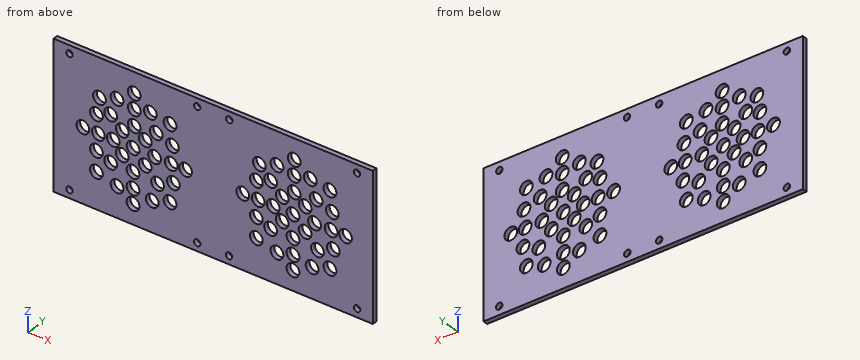
```python
from build123d import *

# Parameters (mm, degrees)
SKETCH1_W           = 200
SKETCH1_H           = 90
BOSS_EXTRUDE1_DEPTH = 3
SKETCH2_R           = 2
SKETCH2_R_2         = 4
CUT_EXTRUDE1_DEPTH  = 3


with BuildPart() as part:
    # Sketch1 → Boss-Extrude1 (new body)
    with BuildSketch(Plane(origin=(0, 0, 0), x_dir=(1, 0, 0), z_dir=(0, 1, 0))):
        with Locations((6.810810811, 7.918918919)):
            Rectangle(SKETCH1_W, SKETCH1_H)
    extrude(amount=BOSS_EXTRUDE1_DEPTH)

    # Sketch2 → Cut-Extrude1 (cut)
    with BuildSketch(Plane(origin=(0, 3, 0), x_dir=(1, 0, 0), z_dir=(0, 1, 0))):
        with Locations(Location((-83.189189189, 47.918918919, 0), (0, 0, 270))):
            Circle(SKETCH2_R)
        with Locations(Location((-83.189189189, -32.081081081, 0), (0, 0, 270))):
            Circle(SKETCH2_R)
        with Locations(Location((-3.189189189, 47.918918919, 0), (0, 0, 270))):
            Circle(SKETCH2_R)
        with Locations(Location((-3.189189189, -32.081081081, 0), (0, 0, 270))):
            Circle(SKETCH2_R)
        with Locations(Location((96.97523931, 47.753811706, 0), (0, 0, 270))):
            Circle(SKETCH2_R)
        with Locations(Location((96.890661701, -31.999841307, 0), (0, 0, 270))):
            Circle(SKETCH2_R)
        with Locations(Location((16.73095992, 47.837679145, 0), (0, 0, 270))):
            Circle(SKETCH2_R)
        with Locations(Location((16.92956487, -32.199971625, 0), (0, 0, 270))):
            Circle(SKETCH2_R)
        with Locations(Location((64.409536285, 15.225493569, 0), (0, 0, 270))):
            Circle(SKETCH2_R_2)
        with Locations(Location((64.458960542, 0.301508961, 0), (0, 0, 270))):
            Circle(SKETCH2_R_2)
        with Locations(Location((72.150575188, 22.957645887, 0), (0, 0, 270))):
            Circle(SKETCH2_R_2)
        with Locations(Location((79.984903702, 30.782980722, 0), (0, 0, 270))):
            Circle(SKETCH2_R_2)
        with Locations(Location((42.782150533, -6.377064303, 0), (0, 0, 270))):
            Circle(SKETCH2_R_2)
        with Locations(Location((35.744744462, -13.406391548, 0), (0, 0, 270))):
            Circle(SKETCH2_R_2)
        with Locations(Location((50.031602385, 0.251885254, 0), (0, 0, 270))):
            Circle(SKETCH2_R_2)
        with Locations(Location((71.328743505, -6.540662674, 0), (0, 0, 270))):
            Circle(SKETCH2_R_2)
        with Locations(Location((56.810810811, 7.918918919, 0), (0, 0, 270))):
            Circle(SKETCH2_R_2)
        with Locations(Location((79.984903702, -15.162031659, 0), (0, 0, 270))):
            Circle(SKETCH2_R_2)
        with Locations(Location((50.031602385, 14.670880058, 0), (0, 0, 270))):
            Circle(SKETCH2_R_2)
        with Locations(Location((42.782150533, 21.891194601, 0), (0, 0, 270))):
            Circle(SKETCH2_R_2)
        with Locations(Location((33.854481941, 30.782980722, 0), (0, 0, 270))):
            Circle(SKETCH2_R_2)
        with Locations(Location((70.286929504, 7.918918919, 0), (0, 0, 270))):
            Circle(SKETCH2_R_2)
        with Locations(Location((80.695917052, 7.918918919, 0), (0, 0, 270))):
            Circle(SKETCH2_R_2)
        with Locations(Location((89.69828466, 7.918918919, 0), (0, 0, 270))):
            Circle(SKETCH2_R_2)
        with Locations(Location((35.027656371, 7.918918919, 0), (0, 0, 270))):
            Circle(SKETCH2_R_2)
        with Locations(Location((44.40512263, 7.918918919, 0), (0, 0, 270))):
            Circle(SKETCH2_R_2)
        with Locations(Location((25.368866125, 7.918918919, 0), (0, 0, 270))):
            Circle(SKETCH2_R_2)
        with Locations(Location((57.533575392, -5.280819839, 0), (0, 0, 270))):
            Circle(SKETCH2_R_2)
        with Locations(Location((57.533575392, -15.162031659, 0), (0, 0, 270))):
            Circle(SKETCH2_R_2)
        with Locations(Location((57.533575392, -24.410851007, 0), (0, 0, 270))):
            Circle(SKETCH2_R_2)
        with Locations(Location((56.810810811, 21.891194601, 0), (0, 0, 270))):
            Circle(SKETCH2_R_2)
        with Locations(Location((56.810810811, 31.666397221, 0), (0, 0, 270))):
            Circle(SKETCH2_R_2)
        with Locations(Location((56.810810811, 40.762539492, 0), (0, 0, 270))):
            Circle(SKETCH2_R_2)
        with Locations(Location((33.854481941, 18.444169796, 0), (0, 0, 270))):
            Circle(SKETCH2_R_2)
        with Locations(Location((46.782150533, 34.292087773, 0), (0, 0, 270))):
            Circle(SKETCH2_R_2)
        with Locations(Location((68.786534903, 34.292087773, 0), (0, 0, 270))):
            Circle(SKETCH2_R_2)
        with Locations(Location((82.102536991, 18.670880058, 0), (0, 0, 270))):
            Circle(SKETCH2_R_2)
        with Locations(Location((81.446114352, -3.030227937, 0), (0, 0, 270))):
            Circle(SKETCH2_R_2)
        with Locations(Location((67.661238952, -17.096427325, 0), (0, 0, 270))):
            Circle(SKETCH2_R_2)
        with Locations(Location((46.782150533, -17.096427325, 0), (0, 0, 270))):
            Circle(SKETCH2_R_2)
        with Locations(Location((33.854481941, -3.030227937, 0), (0, 0, 270))):
            Circle(SKETCH2_R_2)
        with Locations(Location((-35.761406417, 15.18771879, 0), (0, 0, 270))):
            Circle(SKETCH2_R_2)
        with Locations(Location((-35.71198216, 0.263734182, 0), (0, 0, 270))):
            Circle(SKETCH2_R_2)
        with Locations(Location((-28.020367515, 22.919871108, 0), (0, 0, 270))):
            Circle(SKETCH2_R_2)
        with Locations(Location((-20.186039001, 30.745205943, 0), (0, 0, 270))):
            Circle(SKETCH2_R_2)
        with Locations(Location((-57.388792169, -6.414839082, 0), (0, 0, 270))):
            Circle(SKETCH2_R_2)
        with Locations(Location((-64.42619824, -13.444166327, 0), (0, 0, 270))):
            Circle(SKETCH2_R_2)
        with Locations(Location((-50.139340317, 0.214110475, 0), (0, 0, 270))):
            Circle(SKETCH2_R_2)
        with Locations(Location((-28.842199198, -6.578437453, 0), (0, 0, 270))):
            Circle(SKETCH2_R_2)
        with Locations(Location((-43.360131891, 7.88114414, 0), (0, 0, 270))):
            Circle(SKETCH2_R_2)
        with Locations(Location((-20.186039001, -15.199806438, 0), (0, 0, 270))):
            Circle(SKETCH2_R_2)
        with Locations(Location((-50.139340317, 14.633105278, 0), (0, 0, 270))):
            Circle(SKETCH2_R_2)
        with Locations(Location((-57.388792169, 21.853419822, 0), (0, 0, 270))):
            Circle(SKETCH2_R_2)
        with Locations(Location((-66.316460761, 30.745205943, 0), (0, 0, 270))):
            Circle(SKETCH2_R_2)
        with Locations(Location((-29.884013198, 7.88114414, 0), (0, 0, 270))):
            Circle(SKETCH2_R_2)
        with Locations(Location((-19.475025651, 7.88114414, 0), (0, 0, 270))):
            Circle(SKETCH2_R_2)
        with Locations(Location((-10.472658042, 7.88114414, 0), (0, 0, 270))):
            Circle(SKETCH2_R_2)
        with Locations(Location((-65.143286331, 7.88114414, 0), (0, 0, 270))):
            Circle(SKETCH2_R_2)
        with Locations(Location((-55.765820072, 7.88114414, 0), (0, 0, 270))):
            Circle(SKETCH2_R_2)
        with Locations(Location((-74.802076578, 7.88114414, 0), (0, 0, 270))):
            Circle(SKETCH2_R_2)
        with Locations(Location((-42.63736731, -5.318594618, 0), (0, 0, 270))):
            Circle(SKETCH2_R_2)
        with Locations(Location((-42.63736731, -15.199806438, 0), (0, 0, 270))):
            Circle(SKETCH2_R_2)
        with Locations(Location((-42.63736731, -24.448625786, 0), (0, 0, 270))):
            Circle(SKETCH2_R_2)
        with Locations(Location((-43.360131891, 21.853419822, 0), (0, 0, 270))):
            Circle(SKETCH2_R_2)
        with Locations(Location((-43.360131891, 31.628622442, 0), (0, 0, 270))):
            Circle(SKETCH2_R_2)
        with Locations(Location((-43.360131891, 40.724764713, 0), (0, 0, 270))):
            Circle(SKETCH2_R_2)
        with Locations(Location((-66.316460761, 18.406395017, 0), (0, 0, 270))):
            Circle(SKETCH2_R_2)
        with Locations(Location((-53.388792169, 34.254312994, 0), (0, 0, 270))):
            Circle(SKETCH2_R_2)
        with Locations(Location((-31.384407799, 34.254312994, 0), (0, 0, 270))):
            Circle(SKETCH2_R_2)
        with Locations(Location((-18.068405712, 18.633105278, 0), (0, 0, 270))):
            Circle(SKETCH2_R_2)
        with Locations(Location((-18.72482835, -3.068002716, 0), (0, 0, 270))):
            Circle(SKETCH2_R_2)
        with Locations(Location((-32.50970375, -17.134202104, 0), (0, 0, 270))):
            Circle(SKETCH2_R_2)
        with Locations(Location((-53.388792169, -17.134202104, 0), (0, 0, 270))):
            Circle(SKETCH2_R_2)
        with Locations(Location((-66.316460761, -3.068002716, 0), (0, 0, 270))):
            Circle(SKETCH2_R_2)
    extrude(amount=-CUT_EXTRUDE1_DEPTH, mode=Mode.SUBTRACT)


solid = part.part
```
Verification items for the finished model (mm, model axes). Give positions to 0.01 mm unless a question says otherwise; leave off trailing zeros. Put each result on its own line as item: value.
Q1. Depth check by flat-ended pin: P1, Ø7, axis at x = 46.78, z = -34.29, coming from the -Y side. Enter the tip coordinate at first touch or a pass-through.
Result:
P1: through
Q2. Scan lines: probe 1 along X at (y, z) = (1.75, -48); probe 2 along Z at (x, y) = (-83.5, 2.2); probe 3 along Z at (x, y) = (74.5, 1.6). Record each from-to range of solid material in increasing order. Write a range as from..to.
Result:
probe 1: -93.19..-85.19, -81.19..-5.19, -1.19..14.74, 18.72..94.99, 98.96..106.81
probe 2: -52.92..-49.89, -45.94..30.11, 34.06..37.08
probe 3: -52.92..-26.19, -19.72..4.1, 8.98..37.08
Q3. Section check A-A on y = 1.9. Count the separate pieces of the cut face and the enclosed holes in it, and give its area (3 significant figures).
Result:
separate pieces: 1
enclosed holes: 74
area: 14,600 mm2
